from build123d import *

# Parameters (mm, degrees)
BOSS_EXTRUDE1_DEPTH = 1.7
FILLET1_R           = 0.5
SKETCH4_W           = 7
SKETCH4_H           = 7
BOSS_EXTRUDE2_DEPTH = 1.15
REVOLVE4_ANGLE      = 180


with BuildPart() as part:
    # Sketch1 → Boss-Extrude1 (new body)
    with BuildSketch(Plane(origin=(0, 0, 0), x_dir=(1, 0, 0), z_dir=(0, 1, 0))):
        with BuildLine():
            Line((6.665114398, -8.355683224), (10.568791137, -1.594316776))
            Line((10.568791137, -1.594316776), (9.365263158, -1.594316776))
            ThreePointArc((9.365263158, -1.594316776), (7.9, 0), (9.365263158, 1.594316776))
            Line((9.365263158, 1.594316776), (10.568791137, 1.594316776))
            Line((10.568791137, 1.594316776), (6.665114398, 8.355683224))
            Line((6.665114398, 8.355683224), (6.063350409, 7.31339742))
            ThreePointArc((6.063350409, 7.31339742), (3.95, 6.84160069), (3.301912749, 8.907714196))
            Line((3.301912749, 8.907714196), (3.903676738, 9.95))
            Line((3.903676738, 9.95), (-3.903676738, 9.95))
            Line((-3.903676738, 9.95), (-3.301912749, 8.907714196))
            ThreePointArc((-3.301912749, 8.907714196), (-3.95, 6.84160069), (-6.063350409, 7.31339742))
            Line((-6.063350409, 7.31339742), (-6.665114398, 8.355683224))
            Line((-6.665114398, 8.355683224), (-10.568791137, 1.594316776))
            Line((-10.568791137, 1.594316776), (-9.365263158, 1.594316776))
            ThreePointArc((-9.365263158, 1.594316776), (-7.9, 0), (-9.365263158, -1.594316776))
            Line((-9.365263158, -1.594316776), (-10.568791137, -1.594316776))
            Line((-10.568791137, -1.594316776), (-6.665114398, -8.355683224))
            Line((-6.665114398, -8.355683224), (-6.063350409, -7.31339742))
            ThreePointArc((-6.063350409, -7.31339742), (-3.95, -6.84160069), (-3.301912749, -8.907714196))
            Line((-3.301912749, -8.907714196), (-3.903676738, -9.95))
            Line((-3.903676738, -9.95), (3.903676738, -9.95))
            Line((3.903676738, -9.95), (3.301912749, -8.907714196))
            ThreePointArc((3.301912749, -8.907714196), (3.95, -6.84160069), (6.063350409, -7.31339742))
            Line((6.063350409, -7.31339742), (6.665114398, -8.355683224))
        make_face()
    extrude(amount=BOSS_EXTRUDE1_DEPTH)

    # Fillet1
    fillet1_edges = [part.edges().sort_by_distance(p)[0] for p in [
        (-6.665114398, 0.85, 8.355683224),
        (-10.568791137, 0.85, 1.594316776),
        (-10.568791137, 0.85, -1.594316776),
        (-6.665114398, 0.85, -8.355683224),
        (-3.903676738, 0.85, -9.95),
        (3.903676738, 0.85, -9.95),
        (6.665114398, 0.85, -8.355683224),
        (10.568791137, 0.85, -1.594316776),
        (10.568791137, 0.85, 1.594316776),
        (6.665114398, 0.85, 8.355683224),
        (3.903676738, 0.85, 9.95),
        (-3.903676738, 0.85, 9.95),
    ]]
    fillet(fillet1_edges, radius=FILLET1_R)

    # Sketch4 → Boss-Extrude2 (add)
    with BuildSketch(Plane(origin=(0, 1.7, 0), x_dir=(1, 0, 0), z_dir=(0, 1, 0))):
        Rectangle(SKETCH4_W, SKETCH4_H)
    extrude(amount=BOSS_EXTRUDE2_DEPTH)

    # Sketch5 → Revolve4 (revolve)
    with BuildSketch(Plane(origin=(0, 2.85, 0), x_dir=(1, 0, 0), z_dir=(0, 1, 0))):
        with BuildLine():
            Line((0, 3.1), (0, -3.1))
            ThreePointArc((0, -3.1), (3.1, 0), (0, 3.1))
        make_face()
    revolve(axis=Axis((0, 2.85, -3.1), (0, 0, 1)), revolution_arc=REVOLVE4_ANGLE)


solid = part.part
Can you work these out from the model? Positions are in its coordinate system, mm. A direction names the side the tool comes from. Coordinates: 2 decimals unless noted, no trailing zeros. Order: outer loops, then holes, each group sorted by start corner. A loop starts at its lowest first (then second) coordinate and runs counter-clockwise, first axis right, second up. Notation, with made-up numbers: (-19, -30.75) - (-13, -30.75) arc R23 ccw to (-13, -2.75) - close; hole circle Ø2 at (33, 14.25). An arc over 180 degrees is marked (long way). Answer as a JSON object with one key per item and string values. Group by question number.
Q1. Will these pins go through, and if not, where does the flat tip stop? P1, Ø1, axis at x = 1, y = 4, coming from the -Z side; P2, Ø0.9, axis at x = 0.5, y = 2.5, coming from the +Z side; P3, Ø1.3, axis at y = 2, z = 0.5, coming from the -X side.
Q2. Imagine slicing it at D-D (x = -0.25). Please give me the cut outline in (y, z), and give its area (3 significant figures).
Q3. We'd pull the mould along X, two halves only. Please class faces 1 (the face through (0, 2, 3.5)), 2 (the face through (-3.5, 2, 0)), 3 (the face through (6.672, 0.862, -7.856)): +X half, -X half, draft (parallel to the pull), parting line (faces both ways), or undercut.
Q4. I need wall thicknesses on line 1 (Y direction, x = 5.25, z = -4); line 2 (X direction, y = 2.3, z = -1.75); line 3 (X direction, y = 0.4, z = 7). Which ranges of each line are inside material? Lowest first, please. Write a range as from..to.
Q5. Imagine slicing it at A-A (z = -7). Please give me the cut outline in (x, y), and give its area (3 significant figures).
Q6. On a 3-axis mill with a long thin cutter (end or side, diameter ignored), from which of +Z, -Z, +X, -X, +Y, -Y can I reach the whole of each face in a straight line? I mean faces 4 (the face through (-3.2, 2.85, -0.8)), 5 (the face through (0, 2, -3.5)), 6 (the face through (3.5, 2, 0)). Say none if no direction works.
Q7. Imagine slicing it at B-B (z = 2). Please give me the cut outline in (x, y).
Q8. Imagine slicing it at C-C (y = 2.15). Please give me the cut outline in (x, z), and give its area (3 significant figures).
Determined:
{
 "1": {"P1": "stops at z = -2.93", "P2": "stops at z = 3.5", "P3": "stops at x = -8.32"},
 "2": {"outline": "(0, -9.95) - (1.7, -9.95) - (1.7, -3.5) - (2.85, -3.5) - (2.85, -3.09) arc R3.09 ccw to (2.85, 3.09) - (2.85, 3.5) - (1.7, 3.5) - (1.7, 9.95) - (0, 9.95) - close", "area": "56.9 mm2"},
 "3": {"face 1": "draft", "face 2": "-X half", "face 3": "undercut"},
 "4": {"line 1": "y = 0..1.7", "line 2": "x = -3.5..3.5", "line 3": "x = -7.45..-5.78, -3.72..3.72, 5.78..7.45"},
 "5": {"outline": "(-7.45, 0) - (-5.78, 0) - (-5.78, 1.7) - (-7.45, 1.7) - close; (-3.72, 0) - (3.72, 0) - (3.72, 1.7) - (-3.72, 1.7) - close; (5.78, 0) - (7.45, 0) - (7.45, 1.7) - (5.78, 1.7) - close", "area": "18.3 mm2"},
 "6": {"face 4": "+Y", "face 5": "-Z, +X, -X, +Y", "face 6": "+Z, -Z, +X, +Y"},
 "7": {"outline": "(-10.19, 0) - (10.19, 0) - (10.19, 1.7) - (3.5, 1.7) - (3.5, 2.85) - (2.37, 2.85) arc R2.37 ccw to (-2.37, 2.85) - (-3.5, 2.85) - (-3.5, 1.7) - (-10.19, 1.7) - close"},
 "8": {"outline": "(-3.5, -3.5) - (3.5, -3.5) - (3.5, 3.5) - (-3.5, 3.5) - close", "area": "49.0 mm2"}
}
